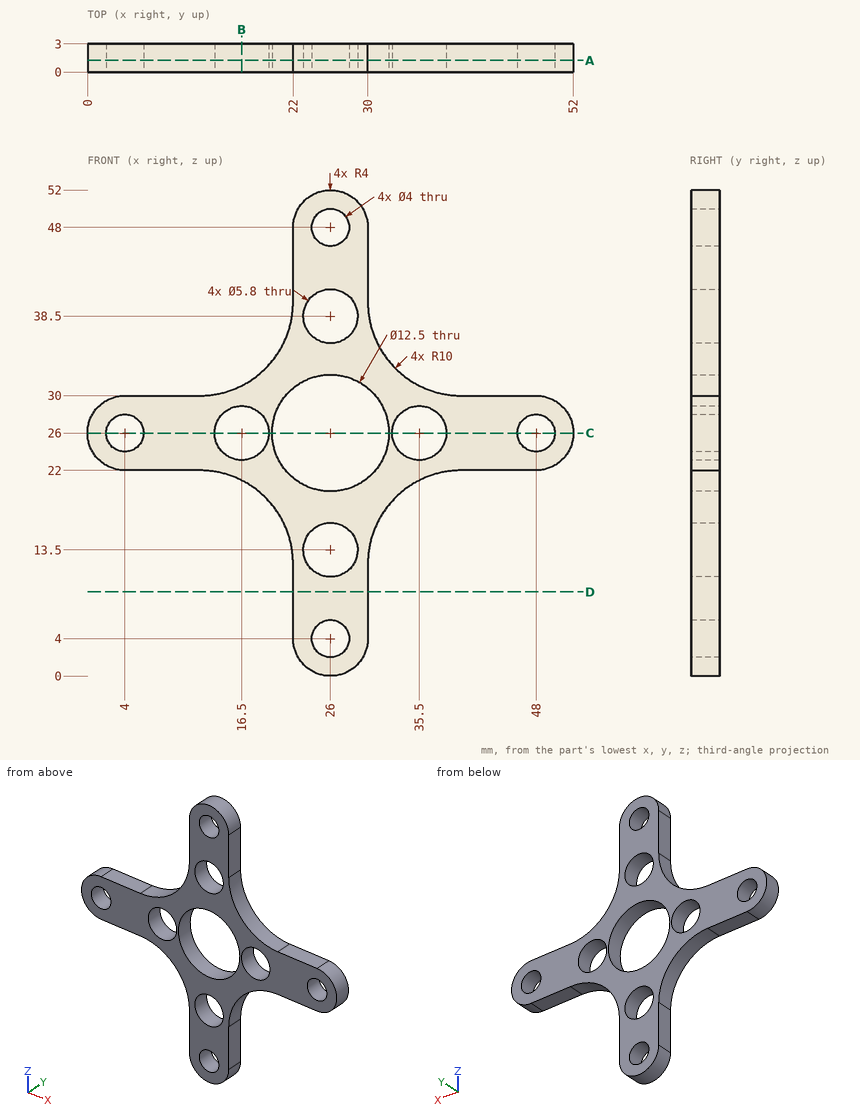
Could you check a few things on this drawing? It's one solid part, dimensions in mm from its lowest x, y, z. Round coordinates to 2 decimals unless told otherwise and drop trailing zeros. Loops run counter-clockwise (first coordinate to the right, second up) from the corner with the lowest first, then second, coordinate; pieces in that order, holes last. Notation, with made-up numbers: (84.25, -2) -> (92.25, -2) arc R20 ccw to (92.25, 9) -> close; hole circle Ø2 at (-32.5, 13.25). An arc over 180 degrees is marked (long way). Answer as CSV lines item,"result".
1. If we section it at C-C on z = 26: Please give me the cut outline in (x, y).
Final values:
outline,"(0, 0) -> (2, 0) -> (2, 3) -> (0, 3) -> close; (6, 0) -> (13.6, 0) -> (13.6, 3) -> (6, 3) -> close; (19.4, 0) -> (19.75, 0) -> (19.75, 3) -> (19.4, 3) -> close; (32.25, 0) -> (32.6, 0) -> (32.6, 3) -> (32.25, 3) -> close; (38.4, 0) -> (46, 0) -> (46, 3) -> (38.4, 3) -> close; (50, 0) -> (52, 0) -> (52, 3) -> (50, 3) -> close"
2. If we section it at A-A on y = 1.25: Count the separate pieces of the cut face and the enclosed holes in it, plus the area to 3 significant figures.
Final values:
separate pieces,"1"
enclosed holes,"9"
area,"548 mm^2"
3. If I drill on L1, parallel to X at y = 2.2, z = 26; L2, parallel to X at y = 1.2, z = 13.5; L3, parallel to Z at x = 8.5, y = 0.6, over which ranges is the centre line in solid material (lowest first)?
Final values:
L1,"x = 0 to 2, 6 to 13.6, 19.4 to 19.75, 32.25 to 32.6, 38.4 to 46, 50 to 52"
L2,"x = 21.89 to 23.1, 28.9 to 30.11"
L3,"z = 22 to 30"
4. If we section it at B-B on x = 16.5: Please give me the cut outline in (y, z).
Final values:
outline,"(0, 20.93) -> (3, 20.93) -> (3, 23.1) -> (0, 23.1) -> close; (0, 28.9) -> (3, 28.9) -> (3, 31.07) -> (0, 31.07) -> close"
5. For pin 1 (3.5 mm diameter, centred on x = 16.5, z = 26, fed in from +Y); pin 2 (1 mm diameter, centred on y = 2, z = 40.5, fed in from +X); pin 3 (0.9 mm diameter, centred on x = 44.5, y = 2, fed in from +Z), each with a flat end and sliding along its axis, tell me the tip position at first contact or that it passes through.
Final values:
pin 1,"passes through"
pin 2,"stops at x = 30"
pin 3,"stops at z = 30"
6. If we section it at D-D on z = 9: Please give me the cut outline in (x, y).
Final values:
outline,"(22, 0) -> (30, 0) -> (30, 3) -> (22, 3) -> close"
